from build123d import *

# Parameters (mm, degrees)
F0_W     = 163.068
F0_H     = 82.804
F1_DEPTH = 9.652
F2_R     = 7.62
F3_R     = 5.08
F4_T     = -2.54


with BuildPart() as f1:
    # F0 (on Top) → F1 (new body)
    with BuildSketch(Plane.XY):
        Rectangle(F0_W, F0_H)
    extrude(amount=F1_DEPTH)

    # F2
    f2_edges = [f1.edges().sort_by_distance(p)[0] for p in [
        (-81.534, 41.402, 4.826),
        (-81.534, -41.402, 4.826),
        (81.534, 41.402, 4.826),
        (81.534, -41.402, 4.826),
    ]]
    fillet(f2_edges, radius=F2_R)

    # F3
    f3_edges = [f1.edges().sort_by_distance(p)[0] for p in [
        (0, -41.402, 9.652),
        (-79.302154, -39.170154, 9.652),
        (79.302154, -39.170154, 9.652),
        (-81.534, 0, 9.652),
        (81.534, 0, 9.652),
        (-79.302154, 39.170154, 9.652),
        (79.302154, 39.170154, 9.652),
        (0, 41.402, 9.652),
    ]]
    fillet(f3_edges, radius=F3_R)

    # F4
    f4_openings = [f1.faces().sort_by_distance(p)[0] for p in [
        (0, 0, 0),
    ]]
    offset(amount=F4_T, openings=f4_openings)


solid = f1.part
Geometry check sheet. Reference: the model listing, model coordinates, mm. A direction names the side the tool comes from. Round coordinates to 2 decimals unless told otherwise and drop trailing zeros. Order: outer loops, then holes, each group sorted by start corner. A loop starts at its lowest first (then second) coordinate and runs counter-clockwise, first axis right, second up. Notation, with made-up numbers: M 32,-33 L 84,-33 A14 ccw 84,-8 Z; hole C 17,48.25 d1. An arc over 180 degrees is marked long. Write each question's results on one line, items separated by ' | '. Start each with the question number.
1. Material ranges on L1, parallel to X at y = 6, z = 2.75; L2, parallel to Y at x = 27.5, z = 1.5; L3, parallel to Z at x = 4, y = -24.5, recorded low to high. Write a range as from..to.
2. Cross-section at C-C on x = 67. Record the boundary of the cut face in (y, z).
3. Cross-section at B-B on y = 11. Record the boundary of the cut face in (x, z), plus the area to 3 significant figures.
4. Cross-section at A-A on z = 3. Record the boundary of the cut face in (x, y).
5. Go/stop test with flat-tipped pins: P1, Ø2, axis at y = 5.5, z = 8.5, coming from the -X side; P2, Ø5, axis at x = -4.5, z = 5.5, coming from the -Y side; P3, Ø4, axis at x = -7, y = -4.5, coming from the -Z side. Record where each tip stops, or that it passes through.
6. Draft check along Y on faces 3 (the face through (1.035, -39.874, 8.203)), 4 (the face through (-1, 1, 9.652)), 5 (the face through (77.47, -37.41, 2.32)), 6 (the face through (-77.55, 37.33, 2.32)). Enter one of: pulls with the +Y half, pulls with the -Y half, needs draft (parallel to the pull), parting line crosses it, or undercut.
7. Set-up check for faces 1 (the face through (-1, 41.402, 2)), 2 (the face through (-78.994, 0, 2)): record each of +Z, -Z, +X, -X, +Y, -Y from which the full face is reachable in a straight line by a thin tool's end or side.
Resolved:
1) L1: -81.53..-78.99, 78.99..81.53 | L2: -41.4..-38.86, 38.86..41.4 | L3: 7.11..9.65
2) outline: M -41.4,0 L -38.86,0 L -38.86,4.57 A2.54 cw -36.32,7.11 L 36.32,7.11 A2.54 cw 38.86,4.57 L 38.86,0 L 41.4,0 L 41.4,4.57 A5.08 ccw 36.32,9.65 L -36.32,9.65 A5.08 ccw -41.4,4.57 Z
3) outline: M -81.53,0 L -78.99,0 L -78.99,4.57 A2.54 cw -76.45,7.11 L 76.45,7.11 A2.54 cw 78.99,4.57 L 78.99,0 L 81.53,0 L 81.53,4.57 A5.08 ccw 76.45,9.65 L -76.45,9.65 A5.08 ccw -81.53,4.57 Z | area: 442 mm2
4) outline: M -81.53,-33.78 A7.62 ccw -73.91,-41.4 L 73.91,-41.4 A7.62 ccw 81.53,-33.78 L 81.53,33.78 A7.62 ccw 73.91,41.4 L -73.91,41.4 A7.62 ccw -81.53,33.78 Z; hole M -78.99,-33.78 A5.08 ccw -73.91,-38.86 L 73.91,-38.86 A5.08 ccw 78.99,-33.78 L 78.99,33.78 A5.08 ccw 73.91,38.86 L -73.91,38.86 A5.08 ccw -78.99,33.78 Z
5) P1: x = -80.61 | P2: y = -41.4 | P3: z = 7.11
6) face 3: pulls with the -Y half | face 4: needs draft | face 5: undercut | face 6: undercut
7) face 1: +Z, -Z, +X, -X, +Y | face 2: -Z
